```python
from build123d import *

# Parameters (mm, degrees)
F0_R          = 5
F0_R_2        = 4
F1_DEPTH      = 25
F2_W          = 21
F2_H          = 21
F3_DEPTH      = 113.501
F3_DEPTH_BACK = 113.501


with BuildPart() as f1:
    # F0 (on Right) → F1 (new body)
    with BuildSketch(Plane.YZ):
        with BuildLine():
            ThreePointArc((101, -12.5), (113.5, 0), (101, 12.5))
            Line((101, 12.5), (-101, 12.5))
            ThreePointArc((-101, 12.5), (-113.5, 0), (-101, -12.5))
            Line((-101, -12.5), (101, -12.5))
        make_face()
        with Locations((-101, 0)):
            Circle(F0_R, mode=Mode.SUBTRACT)
        with Locations((-10, 0)):
            Circle(F0_R_2, mode=Mode.SUBTRACT)
        with Locations((101, 0)):
            Circle(F0_R, mode=Mode.SUBTRACT)
    extrude(amount=F1_DEPTH)

    # F2 (on Front) → F3 (cut, two sides)
    with BuildSketch(Plane.XZ) as f3_sk:
        with Locations((12.5, 0)):
            Rectangle(F2_W, F2_H)
    extrude(amount=-F3_DEPTH, mode=Mode.SUBTRACT)
    extrude(f3_sk.sketch, amount=F3_DEPTH_BACK, mode=Mode.SUBTRACT)


solid = f1.part
```
The listing builds one solid part. Answer for the finished solid, in the listing's coordinates (mm). A direction names the side the tool comes from. Give positions to 0.01 mm unless a question says otherwise; leave off trailing zeros. Order: outer loops, then holes, each group sorted by start corner. A loop starts at its lowest first (then second) coordinate and runs counter-clockwise, first axis right, second up.
1) Find section C-C on z = 0. Give the number of separate pieces and of enclosed holes in the cut face, then the cut area to 3 significant figures.
Reported:
separate pieces: 8
enclosed holes: 0
area: 796 mm2
2) For faces 1 (the face through (12.325, -107.487, -10.685)), 2 (the face through (23, -2, 0)), determine the directions among +Z, -Z, +X, -X, +Y, -Y from which every point of the face is accessible in a straight line to the end or side of a thin tool.
Reported:
face 1: +X, -X, -Y
face 2: +Y, -Y
3) Consider line 1 along Y through (x, z) = (1.1, 0); line 2 along Z through (x, y) = (23.7, -10); line 3 along Z through (x, y) = (23.75, -101). Determine where each line is inside the solid, lowest interval first.
Reported:
line 1: y = -113.5 to -106, -96 to -14, -6 to 96, 106 to 113.5
line 2: z = -12.5 to -4, 4 to 12.5
line 3: z = -12.5 to -5, 5 to 12.5
4) Find section A-A on y = 46.5. Write down the section's boundary in (x, z).
Reported:
outline: (0, -12.5) - (25, -12.5) - (25, 12.5) - (0, 12.5) - close; hole (2, -10.5) - (23, -10.5) - (23, 10.5) - (2, 10.5) - close
5) Find section D-D on y = -10. Write down the section's boundary in (x, z).
Reported:
outline: (0, -12.5) - (25, -12.5) - (25, -4) - (23, -4) - (23, -10.5) - (2, -10.5) - (2, -4) - (0, -4) - close; (0, 4) - (2, 4) - (2, 10.5) - (23, 10.5) - (23, 4) - (25, 4) - (25, 12.5) - (0, 12.5) - close
6) Find section B-B on x = 15.5. Write down the section's boundary in (y, z).
Reported:
outline: (-107.78, -10.5) arc R12.5 ccw to (-101, -12.5) - (101, -12.5) arc R12.5 ccw to (107.78, -10.5) - close; (-107.78, 10.5) - (107.78, 10.5) arc R12.5 ccw to (101, 12.5) - (-101, 12.5) arc R12.5 ccw to start
7) Determine the mould class of faces 3 (the face through (0, -2, 0)), 4 (the face through (12, -1, -12.5)), 5 (the face through (12, -2, -10.5)) for opening direction X: pulls with the +X half, pulls with the -X half, needs draft (parallel to the pull), parting line crosses it, or undercut.
Reported:
face 3: pulls with the -X half
face 4: needs draft
face 5: undercut
8) Given P1, Ø7, axis at y = -10, z = 0, coming from the -X side, flat-ended and moving along its own axis, determine where the tip first touches the part or whether it passes through.
Reported:
P1: passes through
